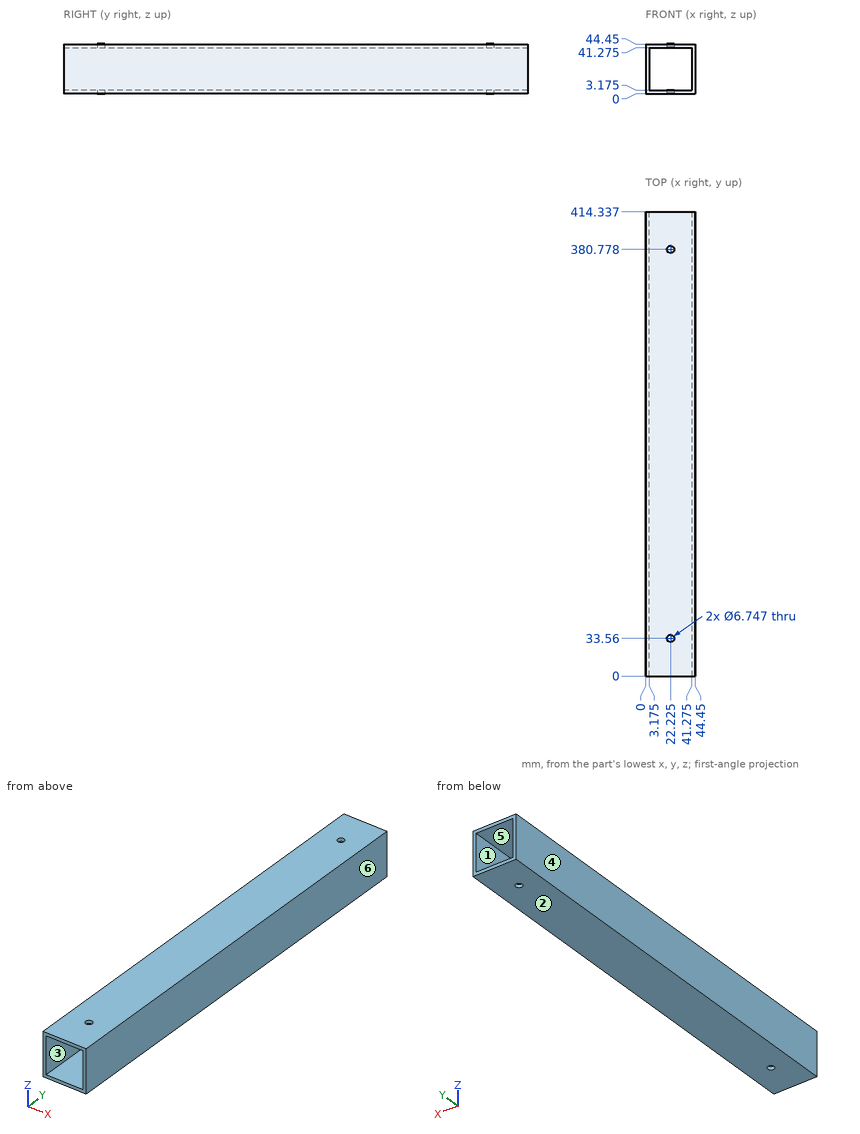
Geometry check sheet. Reference: drawing and pictorial views, mm from the part's lowest x, y, z. A direction names the side the tool comes from. Coordinates: 2 decimals unless noted, no trailing zeros. Write item = value, one per line. Start each with the question number.
1) Mould release check, pull along X, two halves, no side actions. Record for the marked faces 1, 2, 3 and 4: +X half, -X half, draft (parallel to the pull), parting line (faces both ways), or undercut.
2) Material ranges on L1, parallel to Y at x = 23, z = 2 (1 decimal), recorded low to high.
3) Access from +Z, -Z, +X, -X, +Y, -Y to the whole of each face (thin tool, end or side, straight path). Record for the marked faces 5 and 6.
Ans:
q1.face_1 = undercut
q1.face_2 = draft
q1.face_3 = undercut
q1.face_4 = -X half
q2.L1 = 0 to 30.3, 36.8 to 377.5, 384.1 to 414.3
q3.face_5 = +Y, -Y
q3.face_6 = +Z, -Z, +X, +Y, -Y
